The listing builds one solid part. Answer for the finished solid, in the listing's coordinates (mm). Face numbers are marked on the shaded views. A direction names the side the tool comes from. Give positions to 0.01 mm unless a question says otherwise; leave off trailing zeros. Loops run counter-clockwise (first coordinate to the right, second up) from the corner with the lowest first, then second, coordinate; pieces in that order, holes last. Notation, with made-up numbers: M 67.5,30 L 90.5,30 A15 ccw 90.5,47 Z; hole C 31.25,72.5 d7. An arc over 180 degrees is marked long. Return JSON: item names as keys, results as strings.
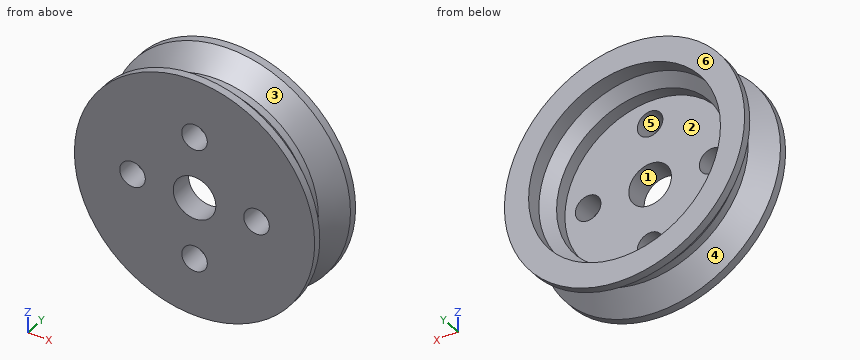
from build123d import *

# Parameters (mm, degrees)
SKETCH_3_R          = 2.75
SKETCH_3_R_2        = 1.65
CUT_EXTRUDE_1_DEPTH = 24.334523779


with BuildPart() as part:
    # Sketch 2 → Revolve 1 (revolve)
    with BuildSketch(Plane.XY, mode=Mode.PRIVATE) as revolve_1_sk:
        Polygon((0, 0), (-15.5, 0), (-15.5, 1), (-13, 3.5), (-13, 4.5), (-15.5, 7), (-15.5, 8), (-12.378679656, 8), (-12.378679656, 6), (-11, 4.621320344), (-11, 3), (0, 3), (0, 1.5), align=None)
    revolve(revolve_1_sk.sketch.rotate(Axis((0, 0, 0), (0, 1, 0)), 180), axis=Axis((0, 0, 0), (0, 1, 0)))

    # Sketch 3 → Cut-Extrude 1 (cut, through all)
    with BuildSketch(Plane.XZ):
        Circle(SKETCH_3_R)
        with Locations((0, 8)):
            Circle(SKETCH_3_R_2)
        with Locations((8, 0)):
            Circle(SKETCH_3_R_2)
        with Locations((0, -8)):
            Circle(SKETCH_3_R_2)
        with Locations((-8, 0)):
            Circle(SKETCH_3_R_2)
    extrude(amount=-CUT_EXTRUDE_1_DEPTH, mode=Mode.SUBTRACT)


solid = part.part
(1) A tool of negligible diameter and unlimited length cuts with its end or side. For the marked faces 1, 2 and 3, from which of +Z, -Z, +X, -X, +Y, -Y can it reach the whole face along a straight path? Write none if from no direction.
Values follow:
{"face 1": "+Y, -Y", "face 2": "+Y", "face 3": "none"}
(2) Straight lines are drawn through the part: line 1 along Z through (x, y) = (0, 2); line 2 along Z through (x, y) = (0, 1.3); line 3 along Z through (x, y) = (0, 7.35). For each, find the intervals that lie inside material, in ascending order.
Values follow:
{"line 1": "-14.5 to -9.65, -6.35 to -2.75, 2.75 to 6.35, 9.65 to 14.5", "line 2": "-15.2 to -9.65, -6.35 to -2.75, 2.75 to 6.35, 9.65 to 15.2", "line 3": "-15.5 to -12.38, 12.38 to 15.5"}
(3) The part is cut by section C-C (y = 6.5). Determine the outline of the cut face in (x, z).
Values follow:
{"outline": "C 0,0 d30; hole C 0,0 d24.76"}
(4) The part is cut by section A-A (z = 0). Give the number of separate pieces and of enclosed holes in the cut face, and give its area (3 significant figures).
Values follow:
{"separate pieces": "4", "enclosed holes": "0", "area": "76.8 mm²"}
(5) Given pin 1 (3 mm diameter, centred on y = 1.5, z = -11, fed in from +X); pin 2 (1 mm diameter, centred on x = 5.5, y = 4.5, fed in from +Z); pin 3 (17.5 mm diameter, centred on x = 0, z = 0, fed in from +Y), each flat-ended and moving along its own axis, determine where each tip first touches the part or whether it passes through.
Values follow:
{"pin 1": "x = 12.18", "pin 2": "z = 12.37", "pin 3": "y = 3"}
(6) Determine the mould class of the marked faces 4, 5 and 6 for opening direction Z: released by +Z, released by -Z, zero draft, split by the parting line, or undercut.
Values follow:
{"face 4": "split by the parting line", "face 5": "undercut", "face 6": "zero draft"}
